Here's how the part is built. I have some questions about the finished solid (model axes, mm). Face numbers are marked on the shaded views. A direction names the side the tool comes from. Round coordinates to 2 decimals unless told otherwise and drop trailing zeros. Loops run counter-clockwise (first coordinate to the right, second up) from the corner with the lowest first, then second, coordinate; pieces in that order, holes last. Notation, with made-up numbers: M -14.5,74 L 29.5,74 A17 cw 29.5,104 Z; hole C 56.5,59.5 d9. An arc over 180 degrees is marked long. Use a Markdown table: item, result.
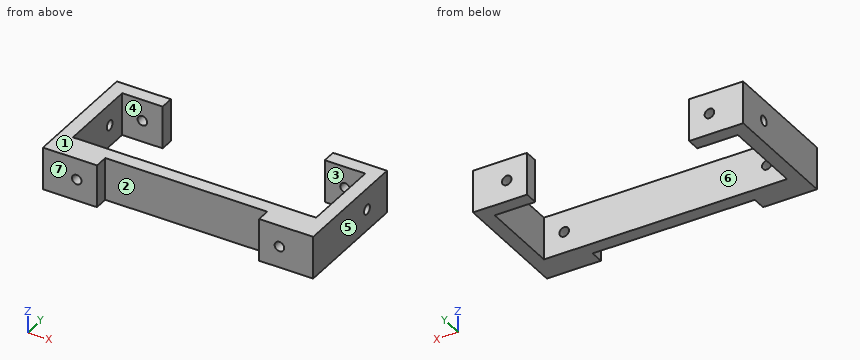
from build123d import *

# Parameters (mm, degrees)
BOSS_EXTRUDE1_DEPTH = 10
CUT_EXTRUDE1_REACH  = 80.154
SKETCH2_R           = 2.25
CUT_EXTRUDE2_REACH  = 130.406
SKETCH3_R           = 2.25
CUT_EXTRUDE3_REACH  = 83.932
SKETCH4_R           = 2.25
CUT_EXTRUDE4_REACH  = 130.406
SKETCH5_R           = 2.25


with BuildPart() as part:
    # Sketch1 → Boss-Extrude1 (new, symmetric)
    with BuildSketch(Plane.XY):
        Polygon((-57.15, -1.651), (-57.15, 36.449), (-38.1, 36.449), (-38.1, 42.799), (-63.5, 42.799), (-63.5, -3.175), (-63.5, -14.351), (-38.1, -14.351), (-38.1, -8.001), (38.1, -8.001), (38.1, -14.351), (63.5, -14.351), (63.5, -3.175), (63.5, 42.799), (38.1, 42.799), (38.1, 36.449), (57.15, 36.449), (57.15, -1.651), align=None)
    extrude(amount=BOSS_EXTRUDE1_DEPTH, both=True)

    # Sketch2 → Cut-Extrude1 (cut, up to next)
    with BuildSketch(Plane(origin=(0, -1.651, 0), x_dir=(1, 0, 0), z_dir=(0, 1, 0)), mode=Mode.PRIVATE) as cut_extrude1_sk1:
        with Locations(Location((-47.625, 0, 0), (0, 0, 270))):
            Circle(SKETCH2_R)
    cut_extrude1_tool1 = extrude(cut_extrude1_sk1.sketch, amount=-CUT_EXTRUDE1_REACH, mode=Mode.PRIVATE) & part.part
    # Sketch2 → Cut-Extrude1 (cut, up to next)
    with BuildSketch(Plane(origin=(0, -1.651, 0), x_dir=(1, 0, 0), z_dir=(0, 1, 0)), mode=Mode.PRIVATE) as cut_extrude1_sk2:
        with Locations(Location((47.625, 0, 0), (0, 0, 180))):
            Circle(SKETCH2_R)
    cut_extrude1_tool2 = extrude(cut_extrude1_sk2.sketch, amount=-CUT_EXTRUDE1_REACH, mode=Mode.PRIVATE) & part.part
    add(cut_extrude1_tool1.solids().sort_by_distance((-47.625, -1.651, 0))[0], mode=Mode.SUBTRACT)
    add(cut_extrude1_tool2.solids().sort_by_distance((47.625, -1.651, 0))[0], mode=Mode.SUBTRACT)

    # Sketch3 → Cut-Extrude2 (cut, up to next)
    with BuildSketch(Plane(origin=(-57.15, 0, 0), x_dir=(0, 0, -1), z_dir=(1, 0, 0)), mode=Mode.PRIVATE) as cut_extrude2_sk1:
        with Locations(Location((0, 26.797, 0), (0, 0, 90))):
            Circle(SKETCH3_R)
    cut_extrude2_tool1 = extrude(cut_extrude2_sk1.sketch, amount=-CUT_EXTRUDE2_REACH, mode=Mode.PRIVATE) & part.part
    add(cut_extrude2_tool1.solids().sort_by_distance((-57.15, 26.797, 0))[0], mode=Mode.SUBTRACT)

    # Sketch4 → Cut-Extrude3 (cut, up to next)
    with BuildSketch(Plane.XZ.offset(-36.449), mode=Mode.PRIVATE) as cut_extrude3_sk1:
        with Locations(Location((-47.625, 0, 0), (0, 0, 90))):
            Circle(SKETCH4_R)
    cut_extrude3_tool1 = extrude(cut_extrude3_sk1.sketch, amount=-CUT_EXTRUDE3_REACH, mode=Mode.PRIVATE) & part.part
    # Sketch4 → Cut-Extrude3 (cut, up to next)
    with BuildSketch(Plane.XZ.offset(-36.449), mode=Mode.PRIVATE) as cut_extrude3_sk2:
        with Locations(Location((47.625, 0, 0), (0, 0, 180))):
            Circle(SKETCH4_R)
    cut_extrude3_tool2 = extrude(cut_extrude3_sk2.sketch, amount=-CUT_EXTRUDE3_REACH, mode=Mode.PRIVATE) & part.part
    add(cut_extrude3_tool1.solids().sort_by_distance((-47.625, 36.449, 0))[0], mode=Mode.SUBTRACT)
    add(cut_extrude3_tool2.solids().sort_by_distance((47.625, 36.449, 0))[0], mode=Mode.SUBTRACT)

    # Sketch5 → Cut-Extrude4 (cut, up to next)
    with BuildSketch(Plane.ZY.offset(-57.15), mode=Mode.PRIVATE) as cut_extrude4_sk1:
        with Locations((0, 27.305)):
            Circle(SKETCH5_R)
    cut_extrude4_tool1 = extrude(cut_extrude4_sk1.sketch, amount=-CUT_EXTRUDE4_REACH, mode=Mode.PRIVATE) & part.part
    add(cut_extrude4_tool1.solids().sort_by_distance((57.15, 27.305, 0))[0], mode=Mode.SUBTRACT)


solid = part.part
1. I need wall thicknesses on probe 1 along Y at (x, z) = (61.5, 0) (3 decimals); probe 2 along X at (y, z) = (7.5, 2.5); probe 3 along Y at (x, z) = (-52.5, 4.5). Which ranges of each line are inside material? Lowest first, please. Write a range as from..to.
Answer sheet:
| item | result |
|---|---|
| probe 1 | -14.351..25.055, 29.555..42.799 |
| probe 2 | -63.5..-57.15, 57.15..63.5 |
| probe 3 | -14.35..-1.65, 36.45..42.8 |
2. We'd pull the mould along X, two halves only. Please class the marked faces 4, 5, 6 and 7: +X half, -X half, draft (parallel to the pull), parting line (faces both ways), or undercut.
Answer sheet:
| item | result |
|---|---|
| face 4 | undercut |
| face 5 | +X half |
| face 6 | undercut |
| face 7 | draft |
3. Imagine slicing it at B-B, the plane z = -5.5. Write out the boundary of the cut face in (x, y).
Answer sheet:
| item | result |
|---|---|
| outline | M -63.5,-14.35 L -38.1,-14.35 L -38.1,-8 L 38.1,-8 L 38.1,-14.35 L 63.5,-14.35 L 63.5,42.8 L 38.1,42.8 L 38.1,36.45 L 57.15,36.45 L 57.15,-1.65 L -57.15,-1.65 L -57.15,36.45 L -38.1,36.45 L -38.1,42.8 L -63.5,42.8 Z |
4. Imagine slicing it at C-C, the plane z = 0. State how many separate pieces and enclosed holes the cut face has, then the cut area to 3 significant figures.
Answer sheet:
| item | result |
|---|---|
| separate pieces | 7 |
| enclosed holes | 0 |
| area | 1,710 mm2 |
5. Which directions (+Z, -Z, +X, -X, +Y, -Y) give clear straight access to the entire face, cutting with the end or side of a thin tool? Please do the marked faces 1, 2 and 3.
Answer sheet:
| item | result |
|---|---|
| face 1 | +Z, +X, -X, +Y, -Y |
| face 2 | +Z, -Z, -Y |
| face 3 | +Z, -Z |
6. For pin 1 Ø10 at (x, z) = (0, 5) entering from +Y, with a flat end and sliding along its axis, tell me the tip position at first contact or that it passes through.
Answer sheet:
| item | result |
|---|---|
| pin 1 | y = -1.65 |
7. Imagine slicing it at A-A, the plane y = 19.5. Write out the boundary of the cut face in (x, z).
Answer sheet:
| item | result |
|---|---|
| outline | M -63.5,-10 L -57.15,-10 L -57.15,10 L -63.5,10 Z; M 57.15,-10 L 63.5,-10 L 63.5,10 L 57.15,10 Z |
